Design review of the part built by this model. Coordinates are the model's own, in mm. A direction names the side the tool comes from. Give positions to 0.01 mm unless a question says otherwise; leave off trailing zeros. Order: outer loops, then holes, each group sorted by start corner. A loop starts at its lowest first (then second) coordinate and runs counter-clockwise, first axis right, second up. Notation, with made-up numbers: (53.5, 88.25) -> (58.5, 88.25) arc R21 ccw to (58.5, 108.25) -> close; hole circle Ø7 at (-22, 74.25). An arc over 180 degrees is marked (long way). Use a Markdown table: item, result. Add a question column.
Solid Edge part; units mm, degrees
sketch "Sketch1" plane through (0, 0, 0) normal (1, 0, 0) x (0, 1, 0)
  circle A0 centre (-5, 6.2) radius 1.5
  line L0 (0, 26.2) -> (0, 0)
  line L1 (0, 0) -> (-35, 0)
  line L2 (-35, 0) -> (-35, 3)
  line L3 (-35, 3) -> (-32, 3)
  line L4 (-32, 3) -> (-32, 23.2)
  line L5 (-32, 23.2) -> (-35, 23.2)
  line L6 (-35, 23.2) -> (-35, 26.2)
  line L7 (-35, 26.2) -> (0, 26.2)
  dimension "D1" = 35
  dimension "D2" = 32
extrude "Protrusion1" add sketch "Sketch1" against normal blind 3
properties material "Acier"
1) Add section D-D (z = 17.25). Give the boundary of the cut face in (x, y), then the cut area to 3 significant figures.
2) The part is to be moulded in two halves that separate along Z. For faces 3 (the flat face through (-1, -35, 25)), 4 (the flat face through (-1, -32, 13)), 5 (the flat face through (-1, -18, 26.2)), 6 (the flat face through (-1, -33, 23.2)), say which applies: +Z half, -Z half, draft (parallel to the pull), parting line (faces both ways), or undercut.
3) Machinability: for faces 1 (the flat face through (-1, -34, 3)), 2 (the flat face through (-1, 0, 13)), which of the approach directions +Z, -Z, +X, -X, +Y, -Y give a long, thin tool a straight path to every point of the face, cutting with its end or side? Answer none if there is none.
4) Add section C-C (x = -0.7). Give the boundary of the cut face in (y, z).
5) Add section B-B (y = -5). Give the boundary of the cut face in (x, z).
6) For L1, parallel to Z at x = -1.1, y = -5; L2, parallel to Y at x = -0.3, z = 6.25; L3, parallel to Y at x = -1.55, z = 14, list the stretches that pass through material, from the lowest coordinate up. Write a range as [from, to].
7) Add section A-A (z = 6.2). Give the boundary of the cut face in (x, y).
8) Insertion check: pin 1 (1 mm diameter, centred on x = -2.5, z = 18.5, fed in from -Y). The pin has a flat end and moves straight along its axis. Give the tip position at first contact, or say it passes through.
Worked answers:
| question | item | result |
|---|---|---|
| 1 | outline | (-3, -32) -> (0, -32) -> (0, 0) -> (-3, 0) -> close |
| 1 | area | 96.0 mm^2 |
| 2 | face 3 | draft |
| 2 | face 4 | undercut |
| 2 | face 5 | +Z half |
| 2 | face 6 | undercut |
| 3 | face 1 | +X, -X, -Y |
| 3 | face 2 | +Z, -Z, +X, -X, +Y |
| 4 | outline | (-35, 0) -> (0, 0) -> (0, 26.2) -> (-35, 26.2) -> (-35, 23.2) -> (-32, 23.2) -> (-32, 3) -> (-35, 3) -> close; hole circle Ø3 at (-5, 6.2) |
| 5 | outline | (-3, 0) -> (0, 0) -> (0, 4.7) -> (-3, 4.7) -> close; (-3, 7.7) -> (0, 7.7) -> (0, 26.2) -> (-3, 26.2) -> close |
| 6 | L1 | [0, 4.7], [7.7, 26.2] |
| 6 | L2 | [-32, -6.5], [-3.5, 0] |
| 6 | L3 | [-32, 0] |
| 7 | outline | (-3, -32) -> (0, -32) -> (0, -6.5) -> (-3, -6.5) -> close; (-3, -3.5) -> (0, -3.5) -> (0, 0) -> (-3, 0) -> close |
| 8 | pin 1 | y = -32 |
